from build123d import *

# Parameters (mm, degrees)
SKETCH1_W                      = 314
SKETCH1_H                      = 114
BOSS_EXTRUDE1_DEPTH            = 3
EDGE_FLANGE1_STRIP_W           = 14
EDGE_FLANGE1_STRIP_H           = 3
EDGE_FLANGE1_STRIP_CUT_DEPTH   = 314
EDGE_FLANGE1_STRIP_2_W         = 14
EDGE_FLANGE1_STRIP_2_H         = 3
EDGE_FLANGE1_STRIP_CUT_2_DEPTH = 314
EDGE_FLANGE1_DEPTH             = 314
EDGE_FLANGE1_BEND_DEPTH        = 314
CUT_EXTRUDE1_REACH             = 171.924
SKETCH16_R                     = 10.5


# Sheet-metal steps are written as plain solids
with BuildPart() as part:
    # Sketch1 → Boss-Extrude1 (new body)
    with BuildSketch(Plane(origin=(0, 0, 0), x_dir=(1, 0, 0), z_dir=(0, 1, 0))):
        Rectangle(SKETCH1_W, SKETCH1_H)
    extrude(amount=BOSS_EXTRUDE1_DEPTH)

    # Edge-Flange1 strip (across the edge) → Edge-Flange1 strip cut (cut)
    with BuildSketch(Plane(origin=(-157, 3, 57), x_dir=(0, 0, -1), z_dir=(1, 0, 0))):
        with Locations((-6, -1.5)):
            Rectangle(EDGE_FLANGE1_STRIP_W, EDGE_FLANGE1_STRIP_H)
    extrude(amount=EDGE_FLANGE1_STRIP_CUT_DEPTH, mode=Mode.SUBTRACT)

    # Edge-Flange1 strip 2 (across the edge) → Edge-Flange1 strip cut 2 (cut)
    with BuildSketch(Plane(origin=(157, 3, -57), x_dir=(0, 0, 1), z_dir=(-1, 0, 0))):
        with Locations((-6, -1.5)):
            Rectangle(EDGE_FLANGE1_STRIP_2_W, EDGE_FLANGE1_STRIP_2_H)
    extrude(amount=EDGE_FLANGE1_STRIP_CUT_2_DEPTH, mode=Mode.SUBTRACT)

    # Edge-Flange1 section (across the edge) → Edge-Flange1 (add)
    with BuildSketch(Plane(origin=(-157, 3, 57), x_dir=(0, 0, -1), z_dir=(1, 0, 0))):
        with BuildLine():
            Line((-3, 1), (-3, 22))
            Line((-3, 22), (0, 22))
            Line((0, 22), (0, 1))
            ThreePointArc((0, 1), (0.292893219, 0.292893219), (1, 0))
            Line((1, 0), (1, -3))
            ThreePointArc((1, -3), (-1.828427125, -1.828427125), (-3, 1))
        make_face()
    extrude(amount=EDGE_FLANGE1_DEPTH)

    # Edge-Flange1 section 2 (across the edge) → Edge-Flange1 bend (add)
    with BuildSketch(Plane(origin=(157, 3, -57), x_dir=(0, 0, 1), z_dir=(-1, 0, 0))):
        with BuildLine():
            Line((-3, 1), (-3, 22))
            Line((-3, 22), (0, 22))
            Line((0, 22), (0, 1))
            ThreePointArc((0, 1), (0.292893219, 0.292893219), (1, 0))
            Line((1, 0), (1, -3))
            ThreePointArc((1, -3), (-1.828427125, -1.828427125), (-3, 1))
        make_face()
    extrude(amount=EDGE_FLANGE1_BEND_DEPTH)

    # Sketch16 → Cut-Extrude1 (cut, up to next)
    with BuildSketch(Plane.XZ, mode=Mode.PRIVATE) as cut_extrude1_sk1:
        with Locations(Location((-137, 40, 0), (0, 0, 270))):
            Circle(SKETCH16_R)
    cut_extrude1_tool1 = extrude(cut_extrude1_sk1.sketch, amount=-CUT_EXTRUDE1_REACH, mode=Mode.PRIVATE) & part.part
    # Sketch16 → Cut-Extrude1 (cut, up to next)
    with BuildSketch(Plane.XZ, mode=Mode.PRIVATE) as cut_extrude1_sk2:
        with Locations(Location((-137, -40, 0), (0, 0, 270))):
            Circle(SKETCH16_R)
    cut_extrude1_tool2 = extrude(cut_extrude1_sk2.sketch, amount=-CUT_EXTRUDE1_REACH, mode=Mode.PRIVATE) & part.part
    # Sketch16 → Cut-Extrude1 (cut, up to next)
    with BuildSketch(Plane.XZ, mode=Mode.PRIVATE) as cut_extrude1_sk3:
        with Locations(Location((137, -40, 0), (0, 0, 270))):
            Circle(SKETCH16_R)
    cut_extrude1_tool3 = extrude(cut_extrude1_sk3.sketch, amount=-CUT_EXTRUDE1_REACH, mode=Mode.PRIVATE) & part.part
    # Sketch16 → Cut-Extrude1 (cut, up to next)
    with BuildSketch(Plane.XZ, mode=Mode.PRIVATE) as cut_extrude1_sk4:
        with Locations(Location((137, 40, 0), (0, 0, 270))):
            Circle(SKETCH16_R)
    cut_extrude1_tool4 = extrude(cut_extrude1_sk4.sketch, amount=-CUT_EXTRUDE1_REACH, mode=Mode.PRIVATE) & part.part
    add(cut_extrude1_tool1.solids().sort_by_distance((-137, 0, 40))[0], mode=Mode.SUBTRACT)
    add(cut_extrude1_tool2.solids().sort_by_distance((-137, 0, -40))[0], mode=Mode.SUBTRACT)
    add(cut_extrude1_tool3.solids().sort_by_distance((137, 0, -40))[0], mode=Mode.SUBTRACT)
    add(cut_extrude1_tool4.solids().sort_by_distance((137, 0, 40))[0], mode=Mode.SUBTRACT)


solid = part.part
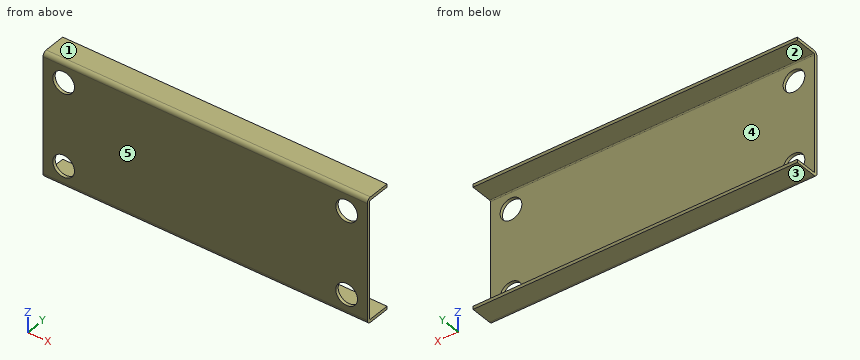
Input: part model. Units: mm. Frame: model coordinates. Face numbers are marked on the shaded views. A direction names the side the tool comes from. Give positions to 0.01 mm unless a question says otherwise; leave off trailing zeros. Order: outer loops, then holes, each group sorted by start corner. A loop starts at its lowest first (then second) coordinate and runs counter-clockwise, first axis right, second up. Notation, with made-up numbers: M 64.5,-27 L 80.5,-27 A14 ccw 80.5,-7 Z; hole C 33.5,47.25 d6. An arc over 180 degrees is marked long. Answer as a JSON object with one key per item and string values.
1. Ray query, line 1 (X direction, y = 2.15, z = 40); line 2 (Z direction, x = 112.5, y = 9.25); line 3 (Y direction, x = -82.5, z = 7). Return the intervals inside material, ascending. Write a range as [from, to].
Result sheet:
{"line 1": "[-157, -147.5], [-126.5, 126.5], [147.5, 157]", "line 2": "[-60, -57], [57, 60]", "line 3": "[0, 3]"}
2. Cut plane C-C, the plane x = 137. Output: boundary loops of the cut face in (y, z), and give its area (3 significant figures).
Result sheet:
{"outline": "M 0,-56 A4 ccw 4,-60 L 25,-60 L 25,-57 L 4,-57 A1 cw 3,-56 L 3,-50.5 L 0,-50.5 Z; M 0,-29.5 L 3,-29.5 L 3,29.5 L 0,29.5 Z; M 0,50.5 L 3,50.5 L 3,56 A1 cw 4,57 L 25,57 L 25,60 L 4,60 A4 ccw 0,56 Z", "area": "360 mm²"}
3. Cut plane D-D, the plane x = -29.5. Output: boundary loops of the cut face in (y, z), and give its area (3 significant figures).
Result sheet:
{"outline": "M 0,-56 A4 ccw 4,-60 L 25,-60 L 25,-57 L 4,-57 A1 cw 3,-56 L 3,56 A1 cw 4,57 L 25,57 L 25,60 L 4,60 A4 ccw 0,56 Z", "area": "486 mm²"}
4. Cut plane A-A, the plane z = 40. Output: boundary loops of the cut face in (x, y), and give its area (3 significant figures).
Result sheet:
{"outline": "M -157,0 L -147.5,0 L -147.5,3 L -157,3 Z; M -126.5,0 L 126.5,0 L 126.5,3 L -126.5,3 Z; M 147.5,0 L 157,0 L 157,3 L 147.5,3 Z", "area": "816 mm²"}
5. Cut plane B-B, the plane y = 8.25. Output: boundary loops of the cut face in (x, z).
Result sheet:
{"outline": "M -157,-60 L 157,-60 L 157,-57 L -157,-57 Z; M -157,57 L 157,57 L 157,60 L -157,60 Z"}
6. Pull-direction query (Z, two-part tool) for the marked faces 1, 2 and 3; classes: +Z half, -Z half, draft (parallel to the pull), parting line (faces both ways), or undercut.
Result sheet:
{"face 1": "+Z half", "face 2": "undercut", "face 3": "-Z half"}
7. First-contact query: P1, Ø2, axis at x = 110.5, z = -0.5, coming from the +Y side. Flat tip, straight axial feed; report the tip coordinate or a pass-through.
Result sheet:
{"P1": "y = 3"}
8. Reachability of the marked faces 4 and 5 from +Z, -Z, +X, -X, +Y, -Y: full face, straight path, thin tool, end or side. Return the list, or none.
Result sheet:
{"face 4": "+X, -X, +Y", "face 5": "+Z, -Z, +X, -X, -Y"}
